from build123d import *

# Parameters (mm, degrees)
BOSS_EXTRU_1_DEPTH   = 3
D_GAGEMENT_M31_D     = 3.4
D_GAGEMENT_M31_DEPTH = 10
D_GAGEMENT_M31_TIP   = 1.021463052


with BuildPart() as part:
    # Esquisse1 → Boss.-Extru.1 (new body)
    with BuildSketch(Plane.XY):
        with BuildLine():
            Line((-5.626876244, 23.692571189), (6.10421614, 33.170262072))
            ThreePointArc((6.10421614, 33.170262072), (7.000718602, 41.608051079), (-1.437070405, 42.504553542))
            Line((-1.437070405, 42.504553542), (-48.270643273, 4.667145735))
            ThreePointArc((-48.270643273, 4.667145735), (-50.15698128, -1.999640667), (-44.5, -6))
            Line((-44.5, -6), (44.5, -6))
            ThreePointArc((44.5, -6), (50.5, 0), (44.5, 6))
            Line((44.5, 6), (3.632012331, 6))
            Line((3.632012331, 6), (-5.626876244, 23.692571189))
        make_face()
        Polygon((-9.91186062, 6), (-15.146064211, 16.001904537), (-27.526006497, 6), align=None, mode=Mode.SUBTRACT)
        with BuildLine():
            ThreePointArc((-3.276233686, 35.233550968), (-3.500359301, 33.124103716), (-1.390912049, 32.8999781))
            Line((-1.390912049, 32.8999781), (3.276233686, 36.670621373))
            ThreePointArc((3.276233686, 36.670621373), (3.500359301, 38.780068625), (1.390912049, 39.00419424))
            Line((1.390912049, 39.00419424), (-3.276233686, 35.233550968))
        make_face(mode=Mode.SUBTRACT)
    extrude(amount=BOSS_EXTRU_1_DEPTH)

    # Dégagement M31
    with Locations(Plane.XY.offset(3)):
        with Locations((-45.329154162, 0.177691477), (-31.329154162, 0.177691477)):
            Hole(D_GAGEMENT_M31_D / 2, depth=D_GAGEMENT_M31_DEPTH)
            with Locations((0, 0, -(D_GAGEMENT_M31_DEPTH + D_GAGEMENT_M31_TIP / 2))):  # 118° drill point
                Cone(0, D_GAGEMENT_M31_D / 2, D_GAGEMENT_M31_TIP, mode=Mode.SUBTRACT)


solid = part.part
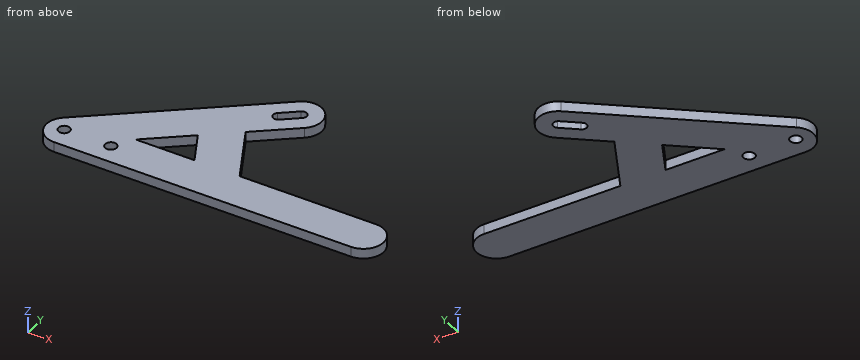
The model under review builds one solid part; all positions refer to its coordinate system, in mm. Round coordinates to 2 decimals unless told otherwise and drop trailing zeros. Write each loop counter-clockwise with the first axis right and the second up, starting at its lowest first coordinate (ties: lowest second). Pieces come first, ordered by that corner, then holes. Notation, with made-up numbers: (-24, 83) - (17, 83) arc R26 cw to (17, 97) - close; hole circle Ø4 at (-25, 46). An arc over 180 degrees is marked (long way). One line per item, written item: value. Start each with the question number.
1. Clearance check with flat-ended pins moving along their axes: P1, Ø0.9, axis at x = -17, z = 1.5, coming from the +Y side; P2, Ø2, axis at x = -31.33, y = 0.18, coming from the -Z side; P3, Ø1.5, axis at x = 22.5, z = 1, coming from the +Y side. State where each tip first meets the part, or that it passes through.
2. Consider section A-A on z = 2.4. Write out the cut boundary in (x, y).
3. Consider section C-C on x = 17.5. Write out the cut boundary in (y, z).
4. Consider section B-B on y = 13. Write out the cut boundary in (x, z), and give its area (3 significant figures).
5. Consider section D-D on y = 20. Write out the cut boundary in (x, z), and give its area (3 significant figures).
6. To check wall thickness, follow L1, parallel to Y at x = -1.5, z = 0.8; L2, parallel to Y at x = 0, z = 0.9; L3, parallel to Y at x = -17, z = 2.25. State the ranges of each line that lie inside material, in increasing order. Write a range as from..to.
Checks:
1. P1: stops at y = 30.29
1. P2: passes through
1. P3: stops at y = 6
2. outline: (-48.27, 4.67) arc R6 ccw to (-44.5, -6) - (44.5, -6) arc R6 ccw to (44.5, 6) - (3.63, 6) - (-5.63, 23.69) - (6.1, 33.17) arc R6 ccw to (-1.44, 42.5) - close; hole circle Ø3.4 at (-45.33, 0.18); hole circle Ø3.4 at (-31.33, 0.18); hole (-27.53, 6) - (-9.91, 6) - (-15.15, 16) - close; hole (-3.28, 35.23) arc R1.5 ccw to (-1.39, 32.9) - (3.28, 36.67) arc R1.5 ccw to (1.39, 39) - close
3. outline: (-6, 0) - (6, 0) - (6, 3) - (-6, 3) - close
4. outline: (-37.96, 0) - (-18.86, 0) - (-18.86, 3) - (-37.96, 3) - close; (-13.58, 0) - (-0.03, 0) - (-0.03, 3) - (-13.58, 3) - close
4. area: 97.9 mm^2
5. outline: (-29.29, 0) - (-3.69, 0) - (-3.69, 3) - (-29.29, 3) - close
5. area: 76.8 mm^2
6. L1: y = -6..15.81, 27.03..32.82, 36.67..42.45
6. L2: y = -6..12.94, 28.24..34.02, 37.88..43.37
6. L3: y = -6..6, 14.5..29.93
